from build123d import *

# Parameters (mm, degrees)
SKETCH1_R           = 15
SKETCH1_R_2         = 1
SKETCH1_R_3         = 1.000000019
SKETCH1_R_4         = 3
BOSS_EXTRUDE1_DEPTH = 5


with BuildPart() as part:
    # Sketch1 → Boss-Extrude1 (new body)
    with BuildSketch(Plane.XY):
        with Locations((-0.041510791, -0.108617644)):
            Circle(SKETCH1_R)
        with Locations((-0.041510791, 11.891382356)):
            Circle(SKETCH1_R_2, mode=Mode.SUBTRACT)
        with Locations((8.443770584, 8.37666373)):
            Circle(SKETCH1_R_2, mode=Mode.SUBTRACT)
        with Locations((11.958489209, -0.108617664)):
            Circle(SKETCH1_R_3, mode=Mode.SUBTRACT)
        with Locations((-0.041510791, -12.108617644)):
            Circle(SKETCH1_R_2, mode=Mode.SUBTRACT)
        with Locations((8.443770584, -8.593899018)):
            Circle(SKETCH1_R_2, mode=Mode.SUBTRACT)
        with Locations((-8.526792165, -8.593899018)):
            Circle(SKETCH1_R_2, mode=Mode.SUBTRACT)
        with Locations((-12.041510791, -0.108617644)):
            Circle(SKETCH1_R_2, mode=Mode.SUBTRACT)
        with Locations((-8.526792165, 8.37666373)):
            Circle(SKETCH1_R_2, mode=Mode.SUBTRACT)
        with Locations((-0.041510791, -0.108617644)):
            Circle(SKETCH1_R_4, mode=Mode.SUBTRACT)
    extrude(amount=BOSS_EXTRUDE1_DEPTH)


solid = part.part
Build history of the part. All positions in model axes, mm. Round coordinates to 2 decimals unless told otherwise and drop trailing zeros. Write each loop counter-clockwise with the first axis right and the second up, starting at its lowest first coordinate (ties: lowest second). Pieces come first, ordered by that corner, then holes. Notation, with made-up numbers: (-29, 29) -> (28, 29) arc R29 cw to (28, 49) -> close; hole circle Ø11 at (-30.75, 57). An arc over 180 degrees is marked (long way). Write item = value, one per line.
(1) Probe L1, parallel to X at y = 0, z = 3.35; L2, parallel to Y at x = -0.75, z = 3.9; L3, parallel to X at y = 0.5, z = 1.55. List the from-to ranges inside material, lowest first.
Answer:
L1 = -15.04 to -13.04, -11.05 to -3.04, 2.96 to 10.96, 12.95 to 14.96
L2 = -15.09 to -12.81, -11.4 to -3.02, 2.81 to 11.19, 12.6 to 14.87
L3 = -15.03 to -12.83, -11.25 to -2.98, 2.9 to 11.17, 12.75 to 14.95
(2) Two-plate mould, pull along Y, no slides. Class faces 1 (the face through (-15, 1, 2)), 2 (the face through (-7.99, -7.75, 2.46)), 3 (the face through (-0.3, 3.4, 5)): pulls with the +Y half, pulls with the -Y half, needs draft (parallel to the pull), parting line crosses it, or undercut.
Answer:
face_1 = parting line crosses it
face_2 = undercut
face_3 = needs draft
(3) Band-saw the part on A-A (y = -1.5). Give the cut face in (x, z), then the cut area to 3 significant figures.
Answer:
outline = (-14.98, 0) -> (-2.7, 0) -> (-2.7, 5) -> (-14.98, 5) -> close; (2.62, 0) -> (14.89, 0) -> (14.89, 5) -> (2.62, 5) -> close
area = 123 mm2
(4) Band-saw the part on B-B (x = -9). Give the cut face in (y, z).
Answer:
outline = (-12.14, 0) -> (-9.47, 0) -> (-9.47, 5) -> (-12.14, 5) -> close; (-7.71, 0) -> (7.5, 0) -> (7.5, 5) -> (-7.71, 5) -> close; (9.26, 0) -> (11.92, 0) -> (11.92, 5) -> (9.26, 5) -> close
(5) Band-saw the part on C-C (z = 2.25). State how many separate pieces and enclosed holes the cut face has, then the cut area to 3 significant figures.
Answer:
separate_pieces = 1
enclosed_holes = 9
area = 653 mm2
(6) Flat gauge pins, fed straight in: pin 1 (1.8 mm diameter, centred on x = -8.53, y = 8.38, fed in from +Z); pin 2 (1.5 mm diameter, centred on x = -7.5, z = 4, fed in from -Y). Where does each tip first touch, or does it go through?
Answer:
pin_1 = through
pin_2 = -13.52
(7) Band-saw the part on D-D (x = 2.25). Give the cut face in (y, z).
Answer:
outline = (-14.93, 0) -> (-2.04, 0) -> (-2.04, 5) -> (-14.93, 5) -> close; (1.83, 0) -> (14.72, 0) -> (14.72, 5) -> (1.83, 5) -> close
